Source: CAD feature listing. Evaluate the final solid. Frame: model axes, mm. A direction names the side the tool comes from. Give positions to 0.01 mm unless a question says otherwise; leave off trailing zeros. Use one line per item in the form item = value. Start each with the question number.
(1) First-contact query: P1, Ø1.5, axis at x = -6, y = 6, coming from the +Z side; P2, Ø2, axis at y = 5, z = -1.5, coming from the -X side; P3, Ø5, axis at x = 6, y = 6, coming from the +Z side; P4, Ø3, axis at y = -1, z = -1.5, coming from the -X side. Flat tips, straight axial feed; report the tip coordinate or a pass-through.
(2) Draft query along Y for faces 6 (the face through (3, -2, -5.953)), 7 (the face through (-2.52, -1.93, -2.94)), 8 (the face through (0.014, 5.761, -0.118)). Return one class per face: pulls with the +Y half, pulls with the -Y half, needs draft (parallel to the pull), parting line crosses it, or undercut.
(3) Material intervals for line 1 along Y through (x, z) = (0, -4) (3 decimals); line 2 along X through (y, z) = (0, -3.3) (3 decimals); line 3 along Z through (x, y) = (2.75, -5), sorted ascending. Write a range as from..to.
(4) Set-up query: faces 1 (the face through (6, 0, -3.515)), 2 (the face through (-5.556, 0, -2)), 3 (the face through (2.8, 4.8, -1.7)), 4 (the face through (-4, 4, -5.709)), 5 (the face through (2.739, -4.834, -1.733)). Return all of +Z, -Z, +X, -X, +Y, -Y with unobstructed straight access to the full face (end or side cutting, diameter ignored); none if empty.
from build123d import *

# Parameters (mm, degrees)
EXTRUDE1_DEPTH         = 5.953125
SKETCH13_R             = 7.540625
EXTRUDE3_DEPTH         = 2.4384
SKETCH2_OUTSIDE_W      = 67.282
SKETCH2_OUTSIDE_H      = 67.282
SKETCH2_OUTSIDE_R      = 5.55625
CUT_EXTRUDE1_DEPTH     = 13.213179277
CUT_EXTRUDE1_DRAFT     = -60
SKETCH4_R              = 3.175
CUT_EXTRUDE3_DEPTH     = 13.213179277
CUT_SWEEP1_PITCH       = 1.27
CUT_SWEEP1_HEIGHT      = 7.223125
CUT_SWEEP1_RADIUS      = 3.175
CUT_SWEEP1_START_ANGLE = 90
SKETCH14_OUTSIDE_W     = 21.51
SKETCH14_OUTSIDE_H     = 21.51
SKETCH14_OUTSIDE_R     = 5.461
CUT_EXTRUDE8_DEPTH     = 0.24384


with BuildPart() as part:
    # Sketch1 → Extrude1 (new body)
    with BuildSketch(Plane.XY):
        Polygon((0, 6.415804866), (-5.55625, 3.207902433), (-5.55625, -3.207902433), (0, -6.415804866), (5.55625, -3.207902433), (5.55625, 3.207902433), align=None)
    extrude(amount=-EXTRUDE1_DEPTH)

    # Sketch13 → Extrude3 (add)
    with BuildSketch(Plane(origin=(0, 0, -5.953125), x_dir=(-1, 0, 0), z_dir=(0, 0, -1))):
        Circle(SKETCH13_R)
    extrude(amount=-EXTRUDE3_DEPTH)


with BuildPart() as cut_extrude1_tool:
    # Sketch2 outside → Cut-Extrude1 (with draft: the straight prism first)
    with BuildSketch(Plane.XY):
        Rectangle(SKETCH2_OUTSIDE_W, SKETCH2_OUTSIDE_H)
        Circle(SKETCH2_OUTSIDE_R, mode=Mode.SUBTRACT)
    extrude(amount=-CUT_EXTRUDE1_DEPTH)
    # Cut-Extrude1: the draft: its side faces are tilted about the plane it starts from
    cut_extrude1_sides = [cut_extrude1_tool.faces().sort_by_distance(p)[0] for p in [
        (0, -33.641, -6.606589638),
        (33.641, 0, -6.606589638),
        (0, 33.641, -6.606589638),
        (-33.641, 0, -6.606589638),
        (-5.55625, 0, -6.606589638),
    ]]
    draft(cut_extrude1_sides, Plane.XY, CUT_EXTRUDE1_DRAFT)


with BuildPart() as part_1:
    add(part.part)

    # Cut-Extrude1: cut by cut_extrude1_tool
    add(cut_extrude1_tool.part, mode=Mode.SUBTRACT)

    # Sketch4 → Cut-Extrude3 (cut, through all)
    with BuildSketch(Plane.XY):
        Circle(SKETCH4_R)
    extrude(amount=-CUT_EXTRUDE3_DEPTH, mode=Mode.SUBTRACT)

    # Cut-Sweep1: sweep along a helix
    with BuildLine() as cut_sweep1_path:
        add(Helix(CUT_SWEEP1_PITCH, CUT_SWEEP1_HEIGHT, CUT_SWEEP1_RADIUS, center=(0, 0, 0), direction=(0, 0, -1), mode=Mode.PRIVATE).rotate(Axis((0, 0, 0), (0, 0, -1)), CUT_SWEEP1_START_ANGLE))
    # Sketch9 → Cut-Sweep1 (sweep, cut)
    with BuildSketch(Plane(origin=(0, 0, 0), x_dir=(0, 0, -1), z_dir=(1, 0, 0))):
        Polygon((-0.635, 3.175), (-0.47625, 3.175), (0, 2.350110803), (-1.11125, 2.350110803), align=None)
    sweep(path=cut_sweep1_path.line, is_frenet=True, mode=Mode.SUBTRACT)

    # Cut-Extrude6 cone 1 section (through the dimple's axis) → Cut-Extrude6 (revolve, cut)
    with BuildSketch(Plane(origin=(0, 0, 0), x_dir=(0, -1, 0), z_dir=(1, 0, 0))):
        Polygon((0, 0), (3.429, 0), (0, 3.429), align=None)
    revolve(axis=Axis((0, 0, 0), (0, 0, -1)), mode=Mode.SUBTRACT)

    # Cut-Extrude7 cone 1 section (through the dimple's axis) → Cut-Extrude7 (revolve, cut)
    with BuildSketch(Plane(origin=(0, 0, -5.953125), x_dir=(0, 1, 0), z_dir=(1, 0, 0))):
        Polygon((0, 0), (3.429, 0), (0, 3.429), align=None)
    revolve(axis=Axis((0, 0, -5.953125), (0, 0, 1)), mode=Mode.SUBTRACT)

    # Sketch14 outside → Cut-Extrude8 (cut)
    with BuildSketch(Plane(origin=(0, 0, -5.953125), x_dir=(-1, 0, 0), z_dir=(0, 0, -1))):
        Rectangle(SKETCH14_OUTSIDE_W, SKETCH14_OUTSIDE_H)
        Circle(SKETCH14_OUTSIDE_R, mode=Mode.SUBTRACT)
    extrude(amount=-CUT_EXTRUDE8_DEPTH, mode=Mode.SUBTRACT)


solid = part_1.part
Geometry says:
q1.P1 = through
q1.P2 = -4.18
q1.P3 = -3.51
q1.P4 = -5.56
q2.face_6 = needs draft
q2.face_7 = undercut
q2.face_8 = pulls with the +Y half
q3.line_1 = -7.541..-3.175, 3.175..7.541
q3.line_2 = -5.556..-3.175, 3.175..5.556
q3.line_3 = -5.71..-3.51
q4.face_1 = +Z
q4.face_2 = +Z, -X, +Y, -Y
q4.face_3 = +Z, +X, +Y
q4.face_4 = -Z
q4.face_5 = +Z, +X, -Y
